```python
from build123d import *

# Parameters (mm, degrees)
SKETCH1_R           = 8
BOSS_EXTRUDE1_DEPTH = 2.5
SKETCH2_R           = 7
BOSS_EXTRUDE2_DEPTH = 0.5
FILLET1_R           = 0.5


with BuildPart() as part:
    # Sketch1 → Boss-Extrude1 (new body)
    with BuildSketch(Plane(origin=(0, 0, 0), x_dir=(1, 0, 0), z_dir=(0, 1, 0))):
        with Locations(Location((0, 0, 0), (0, 0, 270))):
            Circle(SKETCH1_R)
    extrude(amount=BOSS_EXTRUDE1_DEPTH)

    # Sketch2 → Boss-Extrude2 (add)
    with BuildSketch(Plane(origin=(0, 2.5, 0), x_dir=(1, 0, 0), z_dir=(0, 1, 0))):
        with Locations(Location((0, 0, 0), (0, 0, 270))):
            Circle(SKETCH2_R)
    extrude(amount=BOSS_EXTRUDE2_DEPTH)

    # Fillet1
    fillet1_edges = [part.edges().sort_by_distance(p)[0] for p in [
        (0, 0, -8),
        (0, 2.5, -8),
        (0, 3, -7),
    ]]
    fillet(fillet1_edges, radius=FILLET1_R - 0.0001)  # a hair under: the kernel refuses the full size


solid = part.part
```
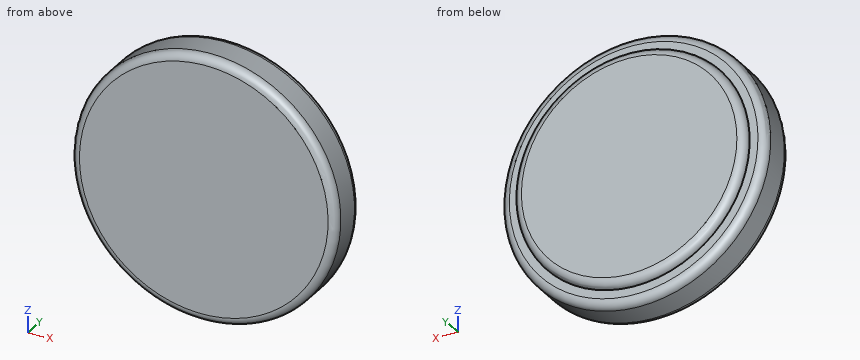
Work out the finished part from the listing and answer in its coordinate system (mm). Give positions to 0.01 mm unless a question says otherwise; leave off trailing zeros. Order: outer loops, then holes, each group sorted by start corner. A loop starts at its lowest first (then second) coordinate and runs counter-clockwise, first axis right, second up. Notation, with made-up numbers: (71, -19) - (87, -19) arc R24 cw to (87, 16) - close; hole circle Ø7 at (-37, -8). An arc over 180 degrees is marked (long way). One line per item, written item: value. Start each with the question number.
1. Section C-C, the plane y = 1.15 is taken. Write down the section's boundary in (x, z).
2. Section D-D, the plane y = 2.7 is taken. Write down the section's boundary in (x, z), then the cut area to 3 significant figures.
3. Consider line 1 (Y direction, x = 7.25, z = 0); line 2 (Z direction, x = -1.75, y = 1.7); line 3 (Z direction, x = -7.25, y = 0.9). Determine where each line is inside the solid, lowest interval first.
Filled sheet:
1. outline: circle Ø16 at (0, 0)
2. outline: circle Ø13.92 at (0, 0)
2. area: 152 mm²
3. line 1: 0 to 2.5
3. line 2: -7.81 to 7.81
3. line 3: -3.38 to 3.38
